Geometry: final body of the model. Coordinates: model frame, mm. Coordinates: 2 decimals unless noted, no trailing zeros. Write each loop counter-clockwise with the first axis right and the second up, starting at its lowest first coordinate (ties: lowest second). Pieces come first, ordered by that corner, then holes. Notation, with made-up numbers: (86, 76.5) -> (93, 76.5) arc R17 cw to (93, 96.5) -> close; hole circle Ø5 at (-38.5, 5). An arc over 180 degrees is marked (long way). One line per item, written item: value.
```python
from build123d import *

# Parameters (mm, degrees)
F1_DEPTH = 30
F2_W     = 70
F2_H     = 30
F3_DEPTH = 30
F4_W     = 95.079931
F4_H     = 30
F5_DEPTH = 30


with BuildPart() as f1:
    # F0 (on Right) → F1 (new body)
    with BuildSketch(Plane.YZ):
        Polygon((133.790882, 890), (31.580462, 890), (-233.790882, -890), (-133.790882, -890), align=None)
    extrude(amount=F1_DEPTH)

    # F2 (on Right) → F3 (cut)
    with BuildSketch(Plane.YZ):
        with Locations((35, 715)):
            Rectangle(F2_W, F2_H)
    extrude(amount=F3_DEPTH, mode=Mode.SUBTRACT)

    # F4 (on Right) → F5 (cut)
    with BuildSketch(Plane.YZ):
        with Locations((-24.192585, 415)):
            Rectangle(F4_W, F4_H)
    extrude(amount=F5_DEPTH, mode=Mode.SUBTRACT)


solid = f1.part
```
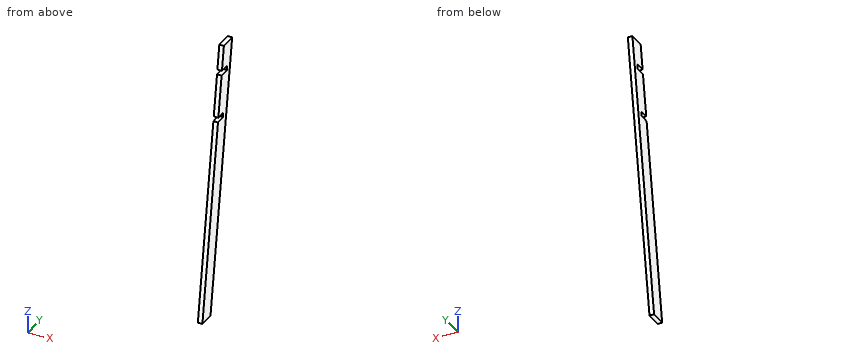
(1) Line query: line 1 (Y direction, x = 11.75, z = -583); line 2 (Y direction, x = 15.25, z = -473). Output: solid intervals per line, ascending. Write a range as [from, to].
Responses:
line 1: y = [-188.02, -87.64]
line 2: y = [-171.62, -71.1]
(2) Section A-A (x = 12.25). Return the cut outline in (y, z).
Responses:
outline: (-233.79, -890) -> (-133.79, -890) -> (133.79, 890) -> (31.58, 890) -> (7.73, 730) -> (70, 730) -> (70, 700) -> (3.25, 700) -> (-37, 430) -> (23.35, 430) -> (23.35, 400) -> (-41.47, 400) -> close
(3) Section B-B (z = -121). Return the cut outline in (x, y).
Responses:
outline: (0, -119.14) -> (30, -119.14) -> (30, -18.19) -> (0, -18.19) -> close
(4) Section C-C (y = -63). Return the cut outline in (x, z).
Responses:
outline: (0, -419.09) -> (30, -419.09) -> (30, 255.59) -> (0, 255.59) -> close
(5) First-contact query: pin 1 (2 mm diameter, centred on x = 12.5, z = 635.5, fed in from -Y); pin 2 (1 mm diameter, centred on x = 17, z = 55, fed in from -Y); pin 3 (15 mm diameter, centred on x = 8, z = 718.5, fed in from -Y). Flat tips, straight axial feed; report the tip coordinate or a pass-through.
Responses:
pin 1: stops at y = -6.51
pin 2: stops at y = -92.98
pin 3: stops at y = 70
